```python
from build123d import *

# Parameters (mm, degrees)
SKETCH1_W           = 120
SKETCH1_H           = 120
BOSS_EXTRUDE1_DEPTH = 3.3
SKETCH2_W           = 10
SKETCH2_H           = 3.3
CUT_EXTRUDE1_DEPTH  = 3.3
LPATTERN1_COUNT     = 5
LPATTERN1_PITCH     = 20
SKETCH3_W           = 120
SKETCH3_H           = 30.4
CUT_EXTRUDE2_DEPTH  = 3.3
SKETCH4_W           = 120
SKETCH4_H           = 3.3
CUT_EXTRUDE3_DEPTH  = 35


with BuildPart() as part:
    # Sketch1 → Boss-Extrude1 (new body)
    with BuildSketch(Plane.XY):
        Rectangle(SKETCH1_W, SKETCH1_H)
    extrude(amount=BOSS_EXTRUDE1_DEPTH)

    # Sketch2 → Cut-Extrude1 (cut)
    with BuildSketch(Plane.XY.offset(3.3)):
        with Locations((45, -18.35)):
            Rectangle(SKETCH2_W, SKETCH2_H)
        with Locations((45, 24.95)):
            Rectangle(SKETCH2_W, SKETCH2_H)
    cut_extrude1 = extrude(amount=-CUT_EXTRUDE1_DEPTH, mode=Mode.SUBTRACT)

    # LPattern1: Cut-Extrude1 ×5
    with Locations(*[(-i * LPATTERN1_PITCH, 0, 0) for i in range(1, LPATTERN1_COUNT)]):
        add(cut_extrude1, mode=Mode.SUBTRACT)

    # Sketch3 → Cut-Extrude2 (cut)
    with BuildSketch(Plane(origin=(0, 0, 0), x_dir=(-1, 0, 0), z_dir=(0, 0, -1))):
        with Locations((0, 44.8)):
            Rectangle(SKETCH3_W, SKETCH3_H)
    extrude(amount=-CUT_EXTRUDE2_DEPTH, mode=Mode.SUBTRACT)

    # Sketch4 → Cut-Extrude3 (cut)
    with BuildSketch(Plane.XZ.offset(60)):
        with Locations((0, 1.65)):
            Rectangle(SKETCH4_W, SKETCH4_H)
    extrude(amount=-CUT_EXTRUDE3_DEPTH, mode=Mode.SUBTRACT)


solid = part.part
```
Input: part model. Units: mm. Frame: model coordinates. A direction names the side the tool comes from. Give positions to 0.01 mm unless a question says otherwise; leave off trailing zeros. Put each result on its own line as item: value.
Item 1: Ray query, L1, parallel to X at y = -19, z = 2.95; L2, parallel to Y at x = -31.5, z = 2.35. Return the intervals inside material, ascending. Write a range as from..to.
Found:
L1: x = -60..-40, -30..-20, -10..0, 10..20, 30..40, 50..60
L2: y = -25..-20, -16.7..23.3, 26.6..29.6
Item 2: Contact query for a flat-ended pin moving along its axis: pin 1 (3 mm diameter, centred on x = 2, y = -1, fed in from -Z). Output: stop coordinate, or through.
Found:
pin 1: stops at z = 0
Item 3: Draft query along X for faces 1 (the flat face through (30, -18, 2)), 2 (the flat face through (60, 2, 2)), 3 (the flat face through (-1, 3, 0)). Return one class per face: +X half, -X half, draft (parallel to the pull), parting line (faces both ways), or undercut.
Found:
face 1: undercut
face 2: +X half
face 3: draft
Item 4: Section query A-A, the plane z = 1.75. Count the separate pieces of the cut face and the enclosed holes in it, then the cut area to 3 significant figures.
Found:
separate pieces: 1
enclosed holes: 10
area: 6,220 mm^2
Item 5: Access query for faces 4 (the flat face through (45, 26.6, 2)), 5 (the flat face through (-60, 2, 2)). Directions: +Z, -Z, +X, -X, +Y, -Y. A direction counts if a zero-diameter tool reaches every point of the face in a straight line with its end or side. Return the directions, or none.
Found:
face 4: +Z, -Z
face 5: +Z, -Z, -X, +Y, -Y
